Model file for the job. Use its own axes, mm. A direction names the side the tool comes from. Round coordinates to 2 decimals unless told otherwise and drop trailing zeros. Order: outer loops, then holes, each group sorted by start corner. A loop starts at its lowest first (then second) coordinate and runs counter-clockwise, first axis right, second up. Notation, with made-up numbers: (32, 47.25) -> (37, 47.25) arc R18 ccw to (37, 57.25) -> close; hole circle Ø6 at (21, 4). An arc over 180 degrees is marked (long way). Use CSV: the item, a comma, the result in double quotes.
```python
from build123d import *

# Parameters (mm, degrees)
F0_W      = 254
F0_H      = 158.75
F1_DEPTH  = 12.7
F2_R      = 19.05
F3_DEPTH  = 12.701
F5_D      = 5.1054
F5_DEPTH  = 38.1
F5_TIP    = 1.5338169022
F7_D      = 5.1054
F7_DEPTH  = 38.1
F7_TIP    = 1.5338169022
F9_D      = 9.525
F11_D     = 11.1125
F13_DEPTH = 12.701
F15_DEPTH = 12.701


with BuildPart() as f1:
    # F0 (on Top) → F1 (new body)
    with BuildSketch(Plane.XY):
        with Locations((127, -79.375)):
            Rectangle(F0_W, F0_H)
    extrude(amount=F1_DEPTH)

    # F2 (on face) → F3 (cut, through all)
    with BuildSketch(Plane.XY.offset(12.7)):
        with Locations((127, -79.375)):
            Circle(F2_R)
    extrude(amount=-F3_DEPTH, mode=Mode.SUBTRACT)

    # F5
    with Locations(Plane.YZ.offset(254)):
        with Locations((-28.575, 6.35), (-130.175, 6.35)):
            Hole(F5_D / 2, depth=F5_DEPTH)
            with Locations((0, 0, -(F5_DEPTH + F5_TIP / 2))):  # 118° drill point
                Cone(0, F5_D / 2, F5_TIP, mode=Mode.SUBTRACT)

    # F7
    with Locations(Plane(origin=(0, 0, 0), x_dir=(0, -1, 0), z_dir=(-1, 0, 0))):
        with Locations((28.575, 6.35), (130.175, 6.35)):
            Hole(F7_D / 2, depth=F7_DEPTH)
            with Locations((0, 0, -(F7_DEPTH + F7_TIP / 2))):  # 118° drill point
                Cone(0, F7_D / 2, F7_TIP, mode=Mode.SUBTRACT)

    # F9 (through all)
    with Locations(Plane.XY.offset(12.7)):
        with Locations((76.2, -79.375)):
            Hole(F9_D / 2)

    # F11 (through all)
    with Locations(Plane.XY.offset(12.7)):
        with Locations((185.7375, -79.375)):
            Hole(F11_D / 2)

    # F12 (on face) → F13 (cut, through all)
    with BuildSketch(Plane.XY.offset(12.7)):
        with BuildLine():
            Line((40.3130046014, -44.4888598491), (40.3128856958, -69.849970228))
            ThreePointArc((40.3128856958, -69.849970228), (46.6526663673, -76.1999917768), (53.0128528986, -69.8704088586))
            ThreePointArc((53.0128528986, -69.8704088586), (53.0128856957, -69.85), (53.0128528986, -69.8295911414))
            Line((53.0128528986, -69.8295911414), (53.0128528986, -44.4704088586))
            ThreePointArc((53.0128528986, -44.4704088586), (46.6536601, -38.1000067017), (40.3130046014, -44.4888598491))
        make_face()
    extrude(amount=-F13_DEPTH, mode=Mode.SUBTRACT)

    # F14 (on face) → F15 (cut, through all)
    with BuildSketch(Plane.XY.offset(12.7)):
        with BuildLine():
            Line((53.0230747203, -114.2974009173), (53.0126976141, -88.9443724583))
            ThreePointArc((53.0126976141, -88.9443724583), (46.6952616172, -82.5602611748), (40.3332976057, -88.9))
            Line((40.3332976057, -88.9), (40.3332976057, -113.9398342138))
            Line((40.3332976057, -113.9398342138), (40.3332976057, -114.6601657862))
            ThreePointArc((40.3332976057, -114.6601657862), (46.8545296788, -120.647406895), (53.0230747203, -114.2974009173))
        make_face()
        with BuildLine():
            Line((40.3332976057, -114.6601657862), (40.3332976057, -113.9398342138))
            ThreePointArc((40.3332976057, -113.9398342138), (40.3230752522, -114.3), (40.3332976057, -114.6601657862))
        make_face()
    extrude(amount=-F15_DEPTH, mode=Mode.SUBTRACT)


solid = f1.part
```
Q1. Mould opens along X. For faces 1 (the cylindrical face through (46.835, -82.562, 6.439)), 2 (the flat face through (0, -80, 6)), 3 (the conical face through (214.633, -28.152, 6.483)) say: +X half, -X half, draft (parallel to the pull), parting line (faces both ways), or undercut.
From the geometry:
face 1,"undercut"
face 2,"-X half"
face 3,"+X half"
Q2. Cut at A-A (x = 127). Give the cut face in (y, z) (3 decimals), plus the area to 3 significant figures.
From the geometry:
outline,"(-158.75, 0) -> (-98.425, 0) -> (-98.425, 12.7) -> (-158.75, 12.7) -> close; (-60.325, 0) -> (0, 0) -> (0, 12.7) -> (-60.325, 12.7) -> close"
area,"1,530 mm²"
Q3. Probe line 1 along Y through (x, z) = (28.5, 6.35); line 2 along X through (y, z) = (-53.5, 9.25); line 3 along Y through (x, z) = (76.2, 8.75). List the from-to ranges inside material, lowest first.
From the geometry:
line 1,"y = -158.75 to -132.73, -127.62 to -31.13, -26.02 to 0"
line 2,"x = 0 to 40.31, 53.01 to 254"
line 3,"y = -158.75 to -84.14, -74.61 to 0"
Q4. Pin check, flat tip, straight feed: pin 1 (3 mm diameter, centred on y = -130.175, z = 6.35, fed in from -X). Stop position of the tip, or through.
From the geometry:
pin 1,"stops at x = 38.73"
Q5. Cut at C-C (x = 18.5). Give the cut face in (y, z) (3 decimals).
From the geometry:
outline,"(-158.75, 0) -> (0, 0) -> (0, 12.7) -> (-158.75, 12.7) -> close; hole circle Ø5.105 at (-130.175, 6.35); hole circle Ø5.105 at (-28.575, 6.35)"
Q6. Which spindle directions (+Z, -Z, +X, -X, +Y, -Y) get a long thin tool onto all of the face, cutting with end or side? Do faces 4 (the flat face through (125, -158.75, 6)), 5 (the cylindrical face through (19.32, -127.82, 5.37)), 6 (the cylindrical face through (234.68, -132.61, 7.12)), 7 (the flat face through (40.333, -101, 6)). Say none if no direction does.
From the geometry:
face 4,"+Z, -Z, +X, -X, -Y"
face 5,"-X"
face 6,"+X"
face 7,"+Z, -Z"
Q7. Cut at B-B (y = -101). Give the cut face in (x, z).
From the geometry:
outline,"(0, 0) -> (40.33, 0) -> (40.33, 12.7) -> (0, 12.7) -> close; (53.02, 0) -> (254, 0) -> (254, 12.7) -> (53.02, 12.7) -> close"
